Model file for the job. Use its own axes, mm. Coordinates: 2 decimals unless noted, no trailing zeros. Order: outer loops, then holes, each group sorted by start corner. A loop starts at its lowest first (then second) coordinate and runs counter-clockwise, first axis right, second up. Notation, with made-up numbers: (34, -31) - (90, -31) arc R14 cw to (90, -21) - close; hole circle Ø11 at (-11, -26). An arc over 180 degrees is marked (long way). Put each result on its own line as item: value. Start each with the question number.
```python
from build123d import *

# Parameters (mm, degrees)
F0_R        = 9
F1_DEPTH    = 8
F2_R        = 8.1
F3_DEPTH    = 10
F4_S5_R     = 8.1
F4_T6_DEPTH = 14
F5_R        = 2.5
F6_DEPTH    = 18.001


# Not quite as in the source:
# - a fillet or chamfer that OpenCascade refuses, or shapes differently, is made with other operations: its cross-section is extruded or revolved along the edge and cut away or added


with BuildPart() as f1:
    # F0 (on Front) → F1 (new body)
    with BuildSketch(Plane.XZ):
        Circle(F0_R)
    extrude(amount=F1_DEPTH)

    # F2 (on face) → F3 (join)
    with BuildSketch(Plane.XZ.offset(8)):
        Circle(F2_R)
    extrude(amount=F3_DEPTH)

    # F4: chamfer of 1 on 1 edges, made by hand


with BuildPart() as f4_tool2:
    # F4_s3 → F4_t4 (revolve)
    with BuildSketch(Plane.XY):
        Polygon((9, -7), (8, -8), (9, -8), align=None)
    revolve(axis=Axis((0, -8, 0), (0, -1, 0)))

    # F4_s5 → F4_t6 (cut, symmetric)
    with BuildSketch(Plane.XZ.offset(7.5)):
        Circle(F4_S5_R)
    extrude(amount=F4_T6_DEPTH, both=True, mode=Mode.SUBTRACT)


with BuildPart() as f1_1:
    add(f1.part)

    # F4_t1: cut F4_tool2
    add(f4_tool2.part, mode=Mode.SUBTRACT)

    # F5 (on face) → F6 (cut, through all)
    with BuildSketch(Plane.XZ.offset(18)):
        Circle(F5_R)
    extrude(amount=-F6_DEPTH, mode=Mode.SUBTRACT)


solid = f1_1.part
```
Item 1: Slice it at D-D, the plane y = -8.25. Give the cut face in (x, z), plus the area to 3 significant figures.
Item 2: Slice it at C-C, the plane y = -3.5. Give the cut face in (x, z).
Item 3: Slice it at A-A, the plane z = 0. Give the cut face in (x, y), plus the area to 3 significant figures.
Item 4: Pull direction Z, two halves, no side cores. Call faces 1 (the face through (2, 0, -2)), 2 (the face through (-0.54, -9.13, -2.44)), 3 (the face through (7.726, -13.021, 2.433)): pulls with the +Z half, pulls with the -Z half, needs draft (parallel to the pull), parting line crosses it, or undercut.
Item 5: Wall check: line 1 along Z through (x, y) = (0, -4); line 2 along Z through (x, y) = (0, -8.75); line 3 along X through (y, z) = (-17, 1.5). Give the ranges that are in metal, low to high.
Item 6: Flat gauge pins, fed straight in: pin 1 Ø2 at (x, y) = (4, -8) entering from -Z; pin 2 Ø2 at (x, y) = (0, -11.5) entering from +Z; pin 3 Ø6 at (y, z) = (-15.5, -3.5) entering from +X. Where does each tip first touch, or does it go through?
Item 7: Slice it at B-B, the plane x = 0. Give the cut face in (y, z).
Here are the results:
1. outline: circle Ø16.2 at (0, 0); hole circle Ø5 at (0, 0)
1. area: 186 mm^2
2. outline: circle Ø18 at (0, 0); hole circle Ø5 at (0, 0)
3. outline: (-9, -7) - (-8.1, -7.9) - (-8.1, -18) - (-2.5, -18) - (-2.5, 0) - (-9, 0) - close; (2.5, -18) - (8.1, -18) - (8.1, -7.9) - (9, -7) - (9, 0) - (2.5, 0) - close
3. area: 215 mm^2
4. face 1: needs draft
4. face 2: undercut
4. face 3: parting line crosses it
5. line 1: z = -9 to -2.5, 2.5 to 9
5. line 2: z = -8.1 to -2.5, 2.5 to 8.1
5. line 3: x = -7.96 to -2, 2 to 7.96
6. pin 1: stops at z = -8.16
6. pin 2: stops at z = 8.1
6. pin 3: stops at x = 8.08
7. outline: (-18, -8.1) - (-7.9, -8.1) - (-7, -9) - (0, -9) - (0, -2.5) - (-18, -2.5) - close; (-18, 2.5) - (0, 2.5) - (0, 9) - (-7, 9) - (-7.9, 8.1) - (-18, 8.1) - close
